```python
from build123d import *

# Parameters (mm, degrees)
EXTRUDE_1_DEPTH     = 90
EXTRUDE_1_2_DEPTH   = 90
SKETCH_3_R          = 1.95
CUT_EXTRUDE_1_DEPTH = 92.809803398
SKETCH_5_W          = 25
SKETCH_5_H          = 5
EXTRUDE_2_DEPTH     = 2
SKETCH_6_R          = 3.5
CUT_EXTRUDE_2_DEPTH = 3.5


with BuildPart() as part:
    # Sketch 1 → Extrude 1 (new body)
    with BuildSketch(Plane(origin=(0, 0, 0), x_dir=(0, 0, -1), z_dir=(1, 0, 0))):
        Polygon((-15, 0), (-15, -6.2), (-13.081136552, -10.2), (-1.95, -10.2), (-1.95, -7.2), (-5, -7.2), (-5, 0), align=None)
    extrude(amount=EXTRUDE_1_DEPTH)


with BuildPart() as body_2:
    # Sketch 1 → Extrude 1 2 (new body)
    with BuildSketch(Plane(origin=(0, 0, 0), x_dir=(0, 0, -1), z_dir=(1, 0, 0))):
        Polygon((13.081136552, -10.2), (15, -6.2), (15, 0), (5, 0), (5, -7.2), (1.95, -7.2), (1.95, -10.2), align=None)
    extrude(amount=EXTRUDE_1_2_DEPTH)


with BuildPart() as cut_extrude_1_tool:
    # Sketch 3 → Cut-Extrude 1 (new, through all)
    with BuildSketch(Plane.XZ.offset(10.2)):
        with Locations(Location((15, 12, 0), (0, 0, 270))):
            Circle(SKETCH_3_R)
        with Locations(Location((15, -12, 0), (0, 0, 270))):
            Circle(SKETCH_3_R)
        with Locations(Location((45, -12, 0), (0, 0, 270))):
            Circle(SKETCH_3_R)
        with Locations(Location((75, -12, 0), (0, 0, 270))):
            Circle(SKETCH_3_R)
        with Locations((110, -12)):
            Circle(SKETCH_3_R)
        with Locations((110, 12)):
            Circle(SKETCH_3_R)
        with Locations(Location((75, 12, 0), (0, 0, 270))):
            Circle(SKETCH_3_R)
        with Locations(Location((45, 12, 0), (0, 0, 270))):
            Circle(SKETCH_3_R)
        with BuildLine():
            ThreePointArc((13.377149497, -13.081136552), (15, -13.95), (16.622850503, -13.081136552))
            Line((16.622850503, -13.081136552), (13.377149497, -13.081136552))
        make_face()
        with BuildLine():
            Line((13.377149497, -13.081136552), (16.622850503, -13.081136552))
            ThreePointArc((16.622850503, -13.081136552), (16.866421507, -12.564774963), (16.95, -12))
            ThreePointArc((16.95, -12), (14.435225037, -10.133578493), (13.377149497, -13.081136552))
        make_face()
        with BuildLine():
            ThreePointArc((43.377149497, -13.081136552), (45, -13.95), (46.622850503, -13.081136552))
            Line((46.622850503, -13.081136552), (43.377149497, -13.081136552))
        make_face()
        with BuildLine():
            Line((43.377149497, -13.081136552), (46.622850503, -13.081136552))
            ThreePointArc((46.622850503, -13.081136552), (46.866421507, -12.564774963), (46.95, -12))
            ThreePointArc((46.95, -12), (44.435225037, -10.133578493), (43.377149497, -13.081136552))
        make_face()
        with BuildLine():
            ThreePointArc((76.622850503, -13.081136552), (76.866421507, -12.564774963), (76.95, -12))
            ThreePointArc((76.95, -12), (74.435225037, -10.133578493), (73.377149497, -13.081136552))
            Line((73.377149497, -13.081136552), (76.622850503, -13.081136552))
        make_face()
        with BuildLine():
            Line((76.622850503, -13.081136552), (73.377149497, -13.081136552))
            ThreePointArc((73.377149497, -13.081136552), (75, -13.95), (76.622850503, -13.081136552))
        make_face()
    extrude(amount=-CUT_EXTRUDE_1_DEPTH)


with BuildPart() as part_1:
    add(part.part)

    # Cut-Extrude 1: cut by cut_extrude_1_tool
    add(cut_extrude_1_tool.part, mode=Mode.SUBTRACT)



with BuildPart() as body_2_1:
    add(body_2.part)

    # Cut-Extrude 1: cut by cut_extrude_1_tool
    add(cut_extrude_1_tool.part, mode=Mode.SUBTRACT)


with BuildPart() as part_2:
    add(part_1.part)

    add(body_2_1.part)  # Extrude 2 merges body 2
    # Sketch 5 → Extrude 2 (add, symmetric)
    with BuildSketch(Plane.XY):
        with Locations((77.5, -7.7)):
            Rectangle(SKETCH_5_W, SKETCH_5_H)
    extrude(amount=EXTRUDE_2_DEPTH, both=True)

    # Sketch 6 → Cut-Extrude 2 (cut)
    with BuildSketch(Plane.XZ.offset(10.2)):
        with Locations((15, 12)):
            Circle(SKETCH_6_R)
        with Locations((15, -12)):
            Circle(SKETCH_6_R)
        with Locations((45, 12)):
            Circle(SKETCH_6_R)
        with Locations((75, 12)):
            Circle(SKETCH_6_R)
        with Locations((75, -12)):
            Circle(SKETCH_6_R)
        with Locations((45, -12)):
            Circle(SKETCH_6_R)
    extrude(amount=-CUT_EXTRUDE_2_DEPTH, mode=Mode.SUBTRACT)


solid = part_2.part
```
Build history of the part. All positions in model axes, mm. A direction names the side the tool comes from. Give positions to 0.01 mm unless a question says otherwise; leave off trailing zeros. Order: outer loops, then holes, each group sorted by start corner. A loop starts at its lowest first (then second) coordinate and runs counter-clockwise, first axis right, second up. Notation, with made-up numbers: M 6,75 L 10,75 A20 cw 10,107 Z; hole C 88.25,-19.5 d8. An arc over 180 degrees is marked long. Return JSON: item names as keys, results as strings.
Q1. Band-saw the part on A-A (y = -1.5). Give the cut face in (x, z).
Answer list:
{"outline": "M 0,-15 L 90,-15 L 90,-5 L 0,-5 Z; M 0,5 L 90,5 L 90,15 L 0,15 Z; hole C 15,-12 d3.9; hole C 15,12 d3.9; hole C 45,-12 d3.9; hole C 45,12 d3.9; hole C 75,-12 d3.9; hole C 75,12 d3.9"}
Q2. Flat gauge pins, fed straight in: pin 1 (3 mm diameter, centred on x = 14, z = -11.5, fed in from -Y); pin 2 (3.5 mm diameter, centred on x = 47.5, y = -9.5, fed in from +Z); pin 3 (1.5 mm diameter, centred on x = 44.5, y = -8.5, fed in from +Z). Where does each tip first touch, or does it go through?
Answer list:
{"pin 1": "stops at y = -6.7", "pin 2": "stops at z = 14.25", "pin 3": "stops at z = 8.73"}
Q3. Band-saw the part on C-C (x = 75). Give the cut face in (y, z), then the cut area to 3 significant figures.
Answer list:
{"outline": "M -10.2,-8.5 L -6.7,-8.5 L -6.7,-10.05 L 0,-10.05 L 0,-5 L -7.2,-5 L -7.2,-2 L -5.2,-2 L -5.2,2 L -7.2,2 L -7.2,5 L 0,5 L 0,10.05 L -6.7,10.05 L -6.7,8.5 L -10.2,8.5 Z; M -6.7,-14.76 L -6.2,-15 L 0,-15 L 0,-13.95 L -6.7,-13.95 Z; M -6.7,13.95 L 0,13.95 L 0,15 L -6.2,15 L -6.7,14.76 Z", "area": "144 mm^2"}
Q4. 3-axis set-ups, long thin cutter, end or side, ignore diameter. For faces 5 (the face through (44, -4, 5)), 6 (the face through (0, -5, 10)), 7 (the face through (44.9, -8.5, 8.5)): which of +Z, -Z, +X, -X, +Y, -Y reach the whole face in a straight line?
Answer list:
{"face 5": "+X, -X, +Y", "face 6": "+Z, -Z, -X, +Y, -Y", "face 7": "-Y"}
Q5. Two-plate mould, pull along Z, no slides. Class faces 1 (the face through (14, -6.7, -10)), 2 (the face through (44, -3, -15)), 3 (the face through (76.933, -3.397, 12.254)), 4 (the face through (44, 0, 10)): pulls with the +Z half, pulls with the -Z half, needs draft (parallel to the pull), parting line crosses it, or undercut.
Answer list:
{"face 1": "undercut", "face 2": "pulls with the -Z half", "face 3": "undercut", "face 4": "needs draft"}
Q6. Band-saw the part on D-D (x = 45). Give the cut face in (y, z).
Answer list:
{"outline": "M -10.2,-8.5 L -6.7,-8.5 L -6.7,-10.05 L 0,-10.05 L 0,-5 L -7.2,-5 L -7.2,-1.95 L -10.2,-1.95 Z; M -10.2,1.95 L -7.2,1.95 L -7.2,5 L 0,5 L 0,10.05 L -6.7,10.05 L -6.7,8.5 L -10.2,8.5 Z; M -6.7,-14.76 L -6.2,-15 L 0,-15 L 0,-13.95 L -6.7,-13.95 Z; M -6.7,13.95 L 0,13.95 L 0,15 L -6.2,15 L -6.7,14.76 Z"}
Q7. Wall check: probe 1 along X at (y, z) = (-5, -12); probe 2 along Z at (x, y) = (19, -1.25); probe 3 along X at (y, z) = (-6.75, 10.5). Give the ranges that are in metal, low to high. Write a range as from..to.
Answer list:
{"probe 1": "x = 0..13.05, 16.95..43.05, 46.95..73.05, 76.95..90", "probe 2": "z = -15..-5, 5..15", "probe 3": "x = 0..11.84, 18.16..41.84, 48.16..71.84, 78.16..90"}
Q8. Band-saw the part on B-B (x = 59.5). Give the cut face in (y, z).
Answer list:
{"outline": "M -10.2,-13.08 L -6.2,-15 L 0,-15 L 0,-5 L -7.2,-5 L -7.2,-1.95 L -10.2,-1.95 Z; M -10.2,1.95 L -7.2,1.95 L -7.2,5 L 0,5 L 0,15 L -6.2,15 L -10.2,13.08 Z"}
